from build123d import *

# Parameters (mm, degrees)
BOSS_EXTRUDE1_DEPTH = 19.05
CUT_EXTRUDE1_DEPTH  = 12.7
FILLET1_R           = 2.54


with BuildPart() as part:
    # Sketch1 → Boss-Extrude1 (new body)
    with BuildSketch(Plane(origin=(0, 0, 0), x_dir=(1, 0, 0), z_dir=(0, 1, 0))):
        with BuildLine():
            Line((12.429156122, 80.324059149), (19.666857156, 93.197517293))
            ThreePointArc((19.666857156, 93.197517293), (0, 95.25), (-19.666857156, 93.197517293))
            Line((-19.666857156, 93.197517293), (-12.429156122, 80.324059149))
            ThreePointArc((-12.429156122, 80.324059149), (0, 81.28), (12.429156122, 80.324059149))
        make_face()
    extrude(amount=BOSS_EXTRUDE1_DEPTH)

    # Sketch3 → Cut-Extrude1 (cut)
    with BuildSketch(Plane.XZ):
        with BuildLine():
            Line((-14.416990913, -83.859754788), (-16.722000277, -87.959598292))
            ThreePointArc((-16.722000277, -87.959598292), (0, -89.535), (16.722000277, -87.959598292))
            Line((16.722000277, -87.959598292), (14.416990913, -83.859754788))
            ThreePointArc((14.416990913, -83.859754788), (0, -85.09), (-14.416990913, -83.859754788))
        make_face()
    extrude(amount=-CUT_EXTRUDE1_DEPTH, mode=Mode.SUBTRACT)

    # Fillet1
    fillet1_edges = [part.edges().sort_by_distance(p)[0] for p in [
        (0, 19.05, -81.28),
        (0, 19.05, -95.25),
    ]]
    fillet(fillet1_edges, radius=FILLET1_R)


solid = part.part
CAD build for the part. Positions are in the model's coordinates, mm. A direction names the side the tool comes from. Give positions to 0.01 mm unless a question says otherwise; leave off trailing zeros. Loops run counter-clockwise (first coordinate to the right, second up) from the corner with the lowest first, then second, coordinate; pieces in that order, holes last. Notation, with made-up numbers: M 84.25,26 L 138.25,26 A8 cw 138.25,31 Z; hole C -35.5,34 d5. An arc over 180 degrees is marked long. One line per question, with ' | ' between items. Start each with the question number.
1. Saw through at A-A on y = 10.75. Give the cut face in (x, z) (3 decimals), plus the area to 3 significant figures.
2. Saw through at B-B on x = 0. Give the cut face in (y, z) (3 decimals).
3. Probe L1, parallel to Y at x = 15.5, z = -86.5; L2, parallel to Z at x = -13.5, y = 1; L3, parallel to Z at x = 12.5, y = 2.25. List the from-to ranges inside material, lowest first. Write a range as from..to.
4. Saw through at C-C on y = 13.5. Give the cut face in (x, z).
5. Two-plate mould, pull along X, no slides. Class faces 3 (the face through (0.28, 8.14, -95.25)), 4 (the face through (-0.235, 6.261, -89.535)), 5 (the face through (0, 0, -83)): pulls with the +X half, pulls with the -X half, needs draft (parallel to the pull), parting line crosses it, or undercut.
6. Flat gauge pins, fed straight in: pin 1 (5 mm diameter, centred on y = 15, z = -92.5, fed in from -X); pin 2 (4 mm diameter, centred on x = -2.5, y = 7, fed in from +Z); pin 3 (4 mm diameter, centred on y = 16, z = -82.5, fed in from -X); pin 4 (3 mm diameter, centred on x = 6, z = -87, fed in from -Y). Where does each tip first touch, or does it go through?
7. 3-axis set-ups, long thin cutter, end or side, ignore diameter. For faces 1 (the face through (-0.17, 8.14, -81.28)), 2 (the face through (0.2, 6.26, -85.09)): which of +Z, -Z, +X, -X, +Y, -Y reach the whole face in a straight line?
8. Saw through at D-D on z = -85.75. Give the cut face in (x, y).
Result sheet:
1) outline: M -19.667,-93.198 A95.25 ccw 19.667,-93.198 L 16.722,-87.96 A89.535 cw -16.722,-87.96 Z; M -14.417,-83.86 A85.09 ccw 14.417,-83.86 L 12.429,-80.324 A81.28 cw -12.429,-80.324 Z | area: 312 mm^2
2) outline: M 0,-95.25 L 16.51,-95.25 A2.54 ccw 19.05,-92.71 L 19.05,-83.82 A2.54 ccw 16.51,-81.28 L 0,-81.28 L 0,-85.09 L 12.7,-85.09 L 12.7,-89.535 L 0,-89.535 Z
3) L1: y = 12.7..19.05 | L2: z = -94.29..-88.51, -84.01..-82.23 | L3: z = -94.43..-88.66, -84.17..-80.45
4) outline: M -19.67,-93.2 A95.25 ccw 19.67,-93.2 L 12.43,-80.32 A81.28 cw -12.43,-80.32 Z
5) face 3: parting line crosses it | face 4: undercut | face 5: needs draft
6) pin 1: stops at x = -19.67 | pin 2: stops at z = -81.16 | pin 3: stops at x = -14.78 | pin 4: stops at y = 12.7
7) face 1: +Z, +Y, -Y | face 2: -Y
8) outline: M -15.48,12.7 L 15.48,12.7 L 15.48,19.05 L -15.48,19.05 Z
